Check sheet for the modelled part. Datum: model origin and axes. Units: mm. Face numbers are marked on the shaded views. A direction names the side the tool comes from. Give positions to 0.01 mm unless a question says otherwise; leave off trailing zeros. Order: outer loops, then holes, each group sorted by start corner. A loop starts at its lowest first (then second) coordinate and runs counter-clockwise, first axis right, second up.
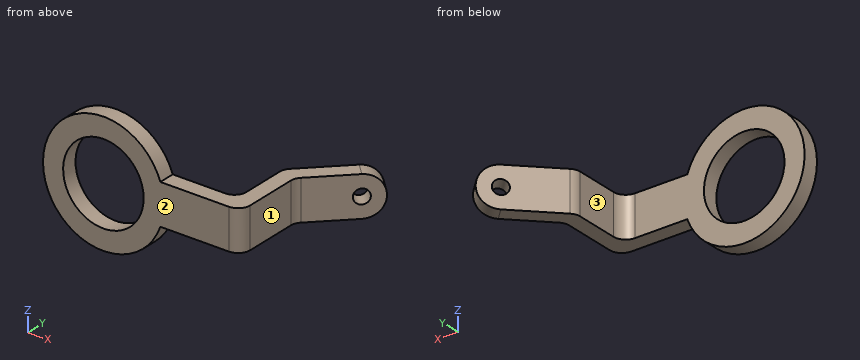
```python
from build123d import *

# Parameters (mm, degrees)
SKETCH2_R            = 10
BOSS_EXTRUDE1_DEPTH  = 4
BOSS_EXTRUDE2_DEPTH  = 10
FILLET1_R            = 5
M3_CLEARANCE_HOLE1_D = 3.6
FILLET2_R            = 3


with BuildPart() as part:
    # Sketch2 → Boss-Extrude1 (new body)
    with BuildSketch(Plane(origin=(0, 0, 0), x_dir=(1, 0, 0), z_dir=(0, 1, 0))):
        with BuildLine():
            Line((34.142135624, 5), (34.142135624, -5))
            Line((34.142135624, -5), (14.142135624, -5))
            ThreePointArc((14.142135624, -5), (-15, 0), (14.142135624, 5))
            Line((14.142135624, 5), (34.142135624, 5))
        make_face()
        with Locations(Location((0, 0, 0), (0, 0, 270))):
            Circle(SKETCH2_R, mode=Mode.SUBTRACT)
    extrude(amount=BOSS_EXTRUDE1_DEPTH)

    # Sketch3 → Boss-Extrude2 (add)
    with BuildSketch(Plane.XY.offset(5)):
        Polygon((34.142135624, 4), (34.142135624, 17.343145751), (47.112698372, 30.313708499), (44.284271247, 33.142135624), (30.142135624, 19), (30.142135624, 4), align=None)
    extrude(amount=-BOSS_EXTRUDE2_DEPTH)

    # Fillet1
    fillet1_edges = [part.edges().sort_by_distance(p)[0] for p in [
        (45.69848481, 31.727922061, 5),
        (45.69848481, 31.727922061, -5),
    ]]
    fillet(fillet1_edges, radius=FILLET1_R - 0.0001)  # a hair under: the kernel refuses the full size

    # M3 Clearance Hole1 (through all)
    with Locations(Plane(origin=(5.571067812, -5.571067812, 0), x_dir=(0.7071067811865489, 0.7071067811865462, 0), z_dir=(-0.7071067811865462, 0.7071067811865489, 0))):
        with Locations((49.748737342, 0)):
            Hole(M3_CLEARANCE_HOLE1_D / 2)

    # Fillet2
    fillet2_edges = [part.edges().sort_by_distance(p)[0] for p in [
        (30.142135624, 4, 0),
        (30.142135624, 19, 0),
        (34.142135624, 17.343145751, 0),
        (34.142135624, 0, 0),
    ]]
    fillet(fillet2_edges, radius=FILLET2_R)


solid = part.part
```
(1) Gauge pin test, flat ends, axial feed: pin 1 Ø3 at (y, z) = (25.5, -2.5) entering from -X; pin 2 Ø1.5 at (x, y) = (34, 17) entering from -Z; pin 3 Ø3 at (y, z) = (8, -1) entering from +X; pin 4 Ø3 at (x, y) = (28.5, 9) entering from +Z. Record the tip position at first contact, or that the pin passes through.
Response values:
pin 1: stops at x = 35.14
pin 2: stops at z = -5
pin 3: stops at x = 34.14
pin 4: passes through
(2) Cross-section at A-A on x = 0. Enter the section's corners in (y, z).
Response values:
outline: (0, -15) - (4, -15) - (4, -10) - (0, -10) - close; (0, 10) - (4, 10) - (4, 15) - (0, 15) - close
(3) Cross-section at C-C on x = 7.5. Enter the section's corners in (y, z).
Response values:
outline: (0, -12.99) - (4, -12.99) - (4, -6.61) - (0, -6.61) - close; (0, 6.61) - (4, 6.61) - (4, 12.99) - (0, 12.99) - close
(4) Set-up check for the marked faces 1, 2 and 3: record each of +Z, -Z, +X, -X, +Y, -Y from which the full face is reachable in a straight line by a thin tool's end or side.
Response values:
face 1: +Z, -Z, +X, -Y
face 2: +Z, -Z, +X, -X, -Y
face 3: +Z, -Z, -X, +Y
(5) Material ranges on L1, parallel to X at y = 2.9, z = 0; L2, parallel to Y at x = 21.5, z = -1; L3, parallel to X at y = 1.3, z = 0, recorded low to high.
Response values:
L1: x = -15 to -10, 10 to 34.14
L2: y = 0 to 4
L3: x = -15 to -10, 10 to 33.61
(6) Cross-section at B-B on y = 15. Enter the section's corners in (x, z).
Response values:
outline: (30.14, -5) - (34.14, -5) - (34.14, 5) - (30.14, 5) - close
